```python
from build123d import *

# Parameters (mm, degrees)
F1_DEPTH = 8


with BuildPart() as f1:
    # F0 (on Top) → F1 (new body)
    with BuildSketch(Plane.XY):
        with BuildLine():
            ThreePointArc((0, 6.968736), (3.636642, 4.340564), (2.5, 0))
            Line((2.5, 0), (2.5, -39.5))
            ThreePointArc((2.5, -39.5), (2.646447, -39.853553), (3, -40))
            Line((3, -40), (3.6, -40))
            ThreePointArc((3.6, -40), (3.953553, -39.853553), (4.1, -39.5))
            Line((4.1, -39.5), (4.1, -37.9))
            Line((4.1, -37.9), (4.1, -36.3))
            Line((4.1, -36.3), (4.1, -34.7))
            Line((4.1, -34.7), (4.1, -33.1))
            Line((4.1, -33.1), (4.1, -31.5))
            Line((4.1, -31.5), (4.1, -29.9))
            Line((4.1, -29.9), (4.1, -28.3))
            Line((4.1, -28.3), (4.1, -26.7))
            Line((4.1, -26.7), (4.1, -25.1))
            Line((4.1, -25.1), (4.1, -23.5))
            Line((4.1, -23.5), (4.1, -21.9))
            Line((4.1, -21.9), (4.1, -20.3))
            Line((4.1, -20.3), (4.1, -18.7))
            Line((4.1, -18.7), (4.1, -17.1))
            Line((4.1, -17.1), (4.1, -15.5))
            Line((4.1, -15.5), (4.1, -0.658339))
            ThreePointArc((4.1, -0.658339), (4.989979, 5.261692), (0, 8.569099))
            Line((0, 8.569099), (0, 6.968736))
        make_face()
        with BuildLine():
            ThreePointArc((-2.5, 0), (-3.636642, 4.340564), (0, 6.968736))
            Line((0, 6.968736), (0, 8.569099))
            ThreePointArc((0, 8.569099), (-4.989979, 5.261692), (-4.1, -0.658339))
            Line((-4.1, -0.658339), (-4.1, -15.5))
            Line((-4.1, -15.5), (-4.1, -17.1))
            Line((-4.1, -17.1), (-4.1, -18.7))
            Line((-4.1, -18.7), (-4.1, -20.3))
            Line((-4.1, -20.3), (-4.1, -21.9))
            Line((-4.1, -21.9), (-4.1, -23.5))
            Line((-4.1, -23.5), (-4.1, -25.1))
            Line((-4.1, -25.1), (-4.1, -26.7))
            Line((-4.1, -26.7), (-4.1, -28.3))
            Line((-4.1, -28.3), (-4.1, -29.9))
            Line((-4.1, -29.9), (-4.1, -31.5))
            Line((-4.1, -31.5), (-4.1, -33.1))
            Line((-4.1, -33.1), (-4.1, -34.7))
            Line((-4.1, -34.7), (-4.1, -36.3))
            Line((-4.1, -36.3), (-4.1, -37.9))
            Line((-4.1, -37.9), (-4.1, -39.5))
            ThreePointArc((-4.1, -39.5), (-3.953553, -39.853553), (-3.6, -40))
            Line((-3.6, -40), (-3, -40))
            ThreePointArc((-3, -40), (-2.646447, -39.853553), (-2.5, -39.5))
            Line((-2.5, -39.5), (-2.5, 0))
        make_face()
        Polygon((4.9, -16.3), (4.1, -15.5), (4.1, -17.1), align=None)
        Polygon((-4.1, -17.1), (-4.1, -15.5), (-4.9, -16.3), align=None)
        Polygon((4.1, -37.9), (4.1, -39.5), (4.9, -38.7), align=None)
        Polygon((4.9, -17.9), (4.1, -17.1), (4.1, -18.7), align=None)
        Polygon((-4.1, -18.7), (-4.1, -17.1), (-4.9, -17.9), align=None)
        Polygon((4.1, -36.3), (4.1, -37.9), (4.9, -37.1), align=None)
        Polygon((4.9, -19.5), (4.1, -18.7), (4.1, -20.3), align=None)
        Polygon((-4.1, -20.3), (-4.1, -18.7), (-4.9, -19.5), align=None)
        Polygon((-4.9, -38.7), (-4.1, -39.5), (-4.1, -37.9), align=None)
        Polygon((4.1, -34.7), (4.1, -36.3), (4.9, -35.5), align=None)
        Polygon((4.9, -21.1), (4.1, -20.3), (4.1, -21.9), align=None)
        Polygon((-4.1, -21.9), (-4.1, -20.3), (-4.9, -21.1), align=None)
        Polygon((-4.9, -37.1), (-4.1, -37.9), (-4.1, -36.3), align=None)
        Polygon((4.1, -33.1), (4.1, -34.7), (4.9, -33.9), align=None)
        Polygon((4.9, -22.7), (4.1, -21.9), (4.1, -23.5), align=None)
        Polygon((-4.1, -23.5), (-4.1, -21.9), (-4.9, -22.7), align=None)
        Polygon((-4.9, -35.5), (-4.1, -36.3), (-4.1, -34.7), align=None)
        Polygon((4.1, -31.5), (4.1, -33.1), (4.9, -32.3), align=None)
        Polygon((4.9, -24.3), (4.1, -23.5), (4.1, -25.1), align=None)
        Polygon((-4.1, -25.1), (-4.1, -23.5), (-4.9, -24.3), align=None)
        Polygon((-4.9, -33.9), (-4.1, -34.7), (-4.1, -33.1), align=None)
        Polygon((4.1, -29.9), (4.1, -31.5), (4.9, -30.7), align=None)
        Polygon((4.9, -25.9), (4.1, -25.1), (4.1, -26.7), align=None)
        Polygon((-4.1, -26.7), (-4.1, -25.1), (-4.9, -25.9), align=None)
        Polygon((-4.9, -32.3), (-4.1, -33.1), (-4.1, -31.5), align=None)
        Polygon((4.1, -28.3), (4.1, -29.9), (4.9, -29.1), align=None)
        Polygon((4.9, -27.5), (4.1, -26.7), (4.1, -28.3), align=None)
        Polygon((-4.1, -28.3), (-4.1, -26.7), (-4.9, -27.5), align=None)
        Polygon((-4.9, -30.7), (-4.1, -31.5), (-4.1, -29.9), align=None)
        Polygon((-4.1, -29.9), (-4.1, -28.3), (-4.9, -29.1), align=None)
    extrude(amount=F1_DEPTH)


solid = f1.part
```
The model under review builds one solid part; all positions refer to its coordinate system, in mm. A direction names the side the tool comes from. Round coordinates to 2 decimals unless told otherwise and drop trailing zeros. Loops run counter-clockwise (first coordinate to the right, second up) from the corner with the lowest first, then second, coordinate; pieces in that order, holes last. Notation, with made-up numbers: M -26,46.5 L 8,46.5 A17 ccw 8,54.5 Z; hole C 2.25,25.25 d6. An arc over 180 degrees is marked long. Answer as a JSON object with one key per item and string values.
(1) Tool access review of faces 3 (the flat face through (3, -16, 0)), 4 (the flat face through (-4.5, -30.3, 3.9)), 5 (the flat face through (4.1, -8, 4)), 6 (the cylindrical face through (3.614, 4.403, 3.944)): name each direction out of +Z, -Z, +X, -X, +Y, -Y from which nothing blocks a thin tool from reaching the whole face with its end or side.
Resolved:
{"face 3": "-Z, +X, -X, +Y, -Y", "face 4": "+Z, -Z, -X", "face 5": "+Z, -Z, +X", "face 6": "+Z, -Z"}
(2) Take a section at C-C on x = -1.25. Give the boundary of the cut face in (y, z).
Resolved:
{"outline": "M 6.73,0 L 8.4,0 L 8.4,8 L 6.73,8 Z"}
(3) Take a section at B-B on y = 2. Give the boundary of the cut face in (x, z), and give its area (3 significant figures).
Resolved:
{"outline": "M -5.38,0 L -3.74,0 L -3.74,8 L -5.38,8 Z; M 3.74,0 L 5.38,0 L 5.38,8 L 3.74,8 Z", "area": "26.2 mm²"}
(4) Take a section at D-D on x = 1.75. Give the boundary of the cut face in (y, z), and give its area (3 significant figures).
Resolved:
{"outline": "M 6.51,0 L 8.25,0 L 8.25,8 L 6.51,8 Z", "area": "13.9 mm²"}
(5) Take a section at A-A on y = -6. Give the boundary of the cut face in (x, z).
Resolved:
{"outline": "M -4.1,0 L -2.5,0 L -2.5,8 L -4.1,8 Z; M 2.5,0 L 4.1,0 L 4.1,8 L 2.5,8 Z"}
(6) Clearance check with flat-ended pins moving along their axes: P1, Ø1, axis at x = -2, z = 4, coming from the +Y side; P2, Ø4, axis at y = -17.5, z = 3, coming from the -X side; P3, Ø2.5, axis at y = -10, z = 3, coming from the +X side. State where each tip first meets the part, or that it passes through.
Resolved:
{"P1": "y = 8.34", "P2": "x = -4.9", "P3": "x = 4.1"}
(7) To check wall thickness, follow line 1 along X through (y, z) = (-13.5, 5); line 2 along X through (y, z) = (-28.5, 4.25); line 3 along Y through (x, z) = (3.5, 4). State the ranges of each line that lie inside material, in increasing order.
Resolved:
{"line 1": "-4.1 to -2.5, 2.5 to 4.1", "line 2": "-4.3 to -2.5, 2.5 to 4.3", "line 3": "-40 to 1.33, 4.67 to 7.25"}
(8) Draft analysis for pull direction Y (two halves, no side actions). For faces 1 (the flat face through (3, -16, 8)), 2 (the flat face through (-4.5, -33.5, 3.9)), state which applies: released by +Y, released by -Y, zero draft, split by the parting line, or undercut.
Resolved:
{"face 1": "zero draft", "face 2": "undercut"}
